Geometry check sheet. Reference: the model listing, model coordinates, mm. Face numbers are marked on the shaded views. A direction names the side the tool comes from. Round coordinates to 2 decimals unless told otherwise and drop trailing zeros. Write each loop counter-clockwise with the first axis right and the second up, starting at its lowest first coordinate (ties: lowest second). Pieces come first, ordered by that corner, then holes.
Item 1: Cross-section at D-D (x = -51.5). Enter the section's corners in (y, z).
Item 2: Access from +Z, -Z, +X, -X, +Y, -Y to the whole of each face (thin tool, end or side, straight path). Record for the marked faces 1 and 2.
Item 3: Scan lines: probe 1 along X at (y, z) = (5.75, -4); probe 2 along X at (y, z) = (1.5, -2); probe 3 along Z at (x, y) = (-28.5, 4.25). Record each from-to range of solid material in increasing order.
Item 4: Cross-section at B-B (x = -45). Enter the section's corners in (y, z), then the cut area to 3 significant figures.
Item 5: Depth check by flat-ended pin: P1, Ø1.5, axis at y = 0.5, z = -1.5, coming from the +X side; P2, Ø1, axis at y = 1.5, z = -2.5, coming from the -X side; P3, Ø2, axis at y = 4.5, z = -2.5, coming from the +X side. Enter the tip coordinate at first touch or a pass-through.
Item 6: Cross-section at C-C (z = -2.25). Enter the section's corners in (x, y), then the cut area to 3 significant figures.
Item 7: Cross-section at A-A (y = 3.5). Enter the section's corners in (x, z).
Autodesk Inventor part; units mm, degrees
ref_plane "YZ Plane" through (0, 0, 0) normal (1, 0, 0) x (0, 1, 0)
ref_plane "XZ Plane" through (0, 0, 0) normal (0, 1, 0) x (-1, 0, 0)
ref_plane "XY Plane" through (0, 0, 0) normal (0, 0, 1) x (1, 0, 0)
sketch "Sketch1" plane through (0, 0, 0) normal (0, 1, 0) x (-1, 0, 0)
  line L0 (0, 0) -> (56, 0)
  line L1 (56, 0) -> (54.5, 0)
  line L2 (56, 0) -> (21.359, -20)
  line L3 (56, 0) -> (96, 0) construction
  line L4 (28, 0) -> (28, 5.9969)
  line L5 (0, 0) -> (34.641, -20)
  line L6 (28, 0) -> (28, -6)
  line L7 (28, -6) -> (78, -6)
  line L8 (28, -6) -> (-22, -6)
  line L9 (56, 0) -> (53.4019, -1.5)
  line L10 (53.4019, -1.5) -> (39.2598, -15.6421)
  line L11 (53.4019, -1.5) -> (73.4019, -1.5) construction
  line L12 (2.5981, -1.5) -> (16.7402, -15.6421)
  point P0 (48.9019, -6)
  point P1 (7.0981, -6)
  dimension "d0" = 56
  dimension "d3" = 40
  dimension "d4" = 150
  dimension "d5" = 6
  dimension "d6" = 50
  dimension "d7" = 50
  dimension "d8" = 3
  dimension "d9" = 20
  dimension "d10" = 135
extrude "Extrusion1" add sketch "Sketch1" along normal blind 6 contours L0 L6 L8 L5 | L0 L2 L7 L6 | L5 L8 L12 | L2 L10 L7
chamfer "Chamfer1" distance 2 angle 45 6 edges at (-48.9019, 3, -6) (-51.1519, 6, -3.75) (-51.1519, 0, -3.75) (-4.8481, 0, -3.75) (-7.0981, 3, -6) (-4.8481, 6, -3.75)
chamfer "Chamfer2" distance 2 angle 45 2 edges at (-37.0367, 0, -6) (-37.0367, 6, -6)
properties part number "parallel_bar_long_no_hole_v2"
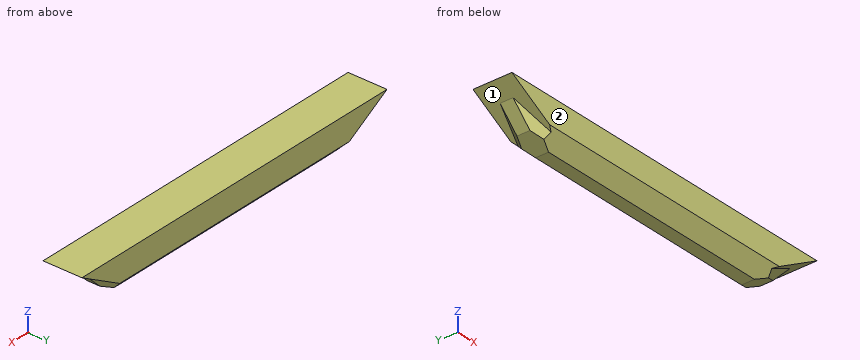
Resolved:
1. outline: (0, -2.6) - (1.43, -2.6) - (2, -3.4) - (4, -3.4) - (4.57, -2.6) - (6, -2.6) - (6, 0) - (0, 0) - close
2. face 1: -Z, -X
2. face 2: +Z, -Z, +X, -X, -Y
3. probe 1: x = -49.07 to -6.93
3. probe 2: x = -52.54 to -3.46
3. probe 3: z = -5.75 to 0
4. outline: (0, -4) - (2, -6) - (4, -6) - (6, -4) - (6, 0) - (0, 0) - close
4. area: 32.0 mm2
5. P1: stops at x = -1.3
5. P2: stops at x = -52.56
5. P3: stops at x = -2.6
6. outline: (-52.65, 2) - (-52.1, 1.61) - (-52.1, 0) - (-3.9, 0) - (-3.9, 1.61) - (-3.35, 2) - (-3.35, 4) - (-3.9, 4.39) - (-3.9, 6) - (-52.1, 6) - (-52.1, 4.39) - (-52.65, 4) - close
6. area: 292 mm2
7. outline: (-56, 0) - (-53.4, -1.5) - (-50.32, -4.59) - (-46.9, -6) - (-9.1, -6) - (-5.68, -4.59) - (-2.6, -1.5) - (0, 0) - close
